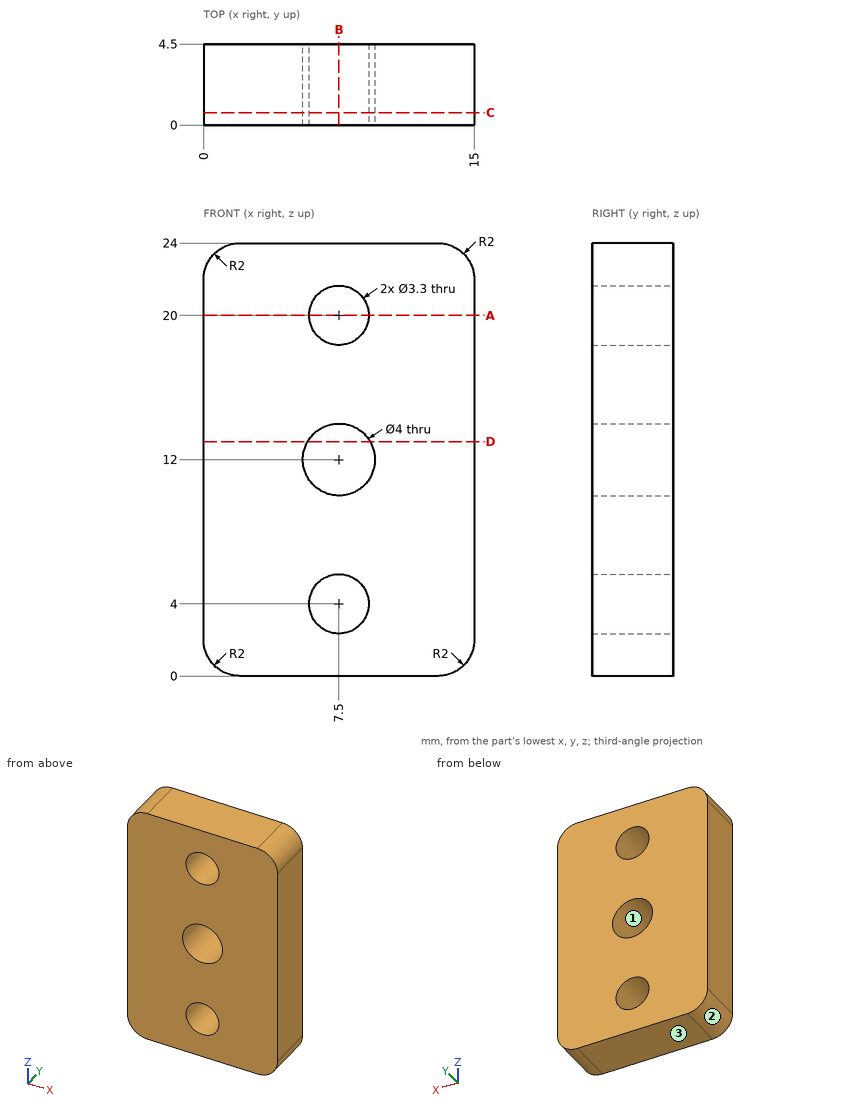
The drawing under review shows one solid part. Ordinate dimensions are in mm from its lowest x, y, z. Coordinates: 2 decimals unless noted, no trailing zeros. Write each loop counter-clockwise with the first axis right and the second up, starting at its lowest first coordinate (ties: lowest second). Pieces come first, ordered by that corner, then holes. Notation, with made-up numbers: (20.25, 71.5) - (50.25, 71.5) arc R17 cw to (50.25, 91.5) - close; hole circle Ø2 at (-11, 59). An arc over 180 degrees is marked (long way). Answer as CSV lines item,"result".
(1) We need section C-C (y = 0.7). Give the boundary of the cut face in (x, z), plus the area to 3 significant figures.
Data:
outline,"(0, 2) arc R2 ccw to (2, 0) - (13, 0) arc R2 ccw to (15, 2) - (15, 22) arc R2 ccw to (13, 24) - (2, 24) arc R2 ccw to (0, 22) - close; hole circle Ø4 at (7.5, 12); hole circle Ø3.3 at (7.5, 4); hole circle Ø3.3 at (7.5, 20)"
area,"327 mm2"
(2) We need section D-D (z = 13). Give the boundary of the cut face in (x, y).
Data:
outline,"(0, 0) - (5.77, 0) - (5.77, 4.5) - (0, 4.5) - close; (9.23, 0) - (15, 0) - (15, 4.5) - (9.23, 4.5) - close"
(3) We need section B-B (x = 7.5). Give the boundary of the cut face in (y, z).
Data:
outline,"(0, 0) - (4.5, 0) - (4.5, 2.35) - (0, 2.35) - close; (0, 5.65) - (4.5, 5.65) - (4.5, 10) - (0, 10) - close; (0, 14) - (4.5, 14) - (4.5, 18.35) - (0, 18.35) - close; (0, 21.65) - (4.5, 21.65) - (4.5, 24) - (0, 24) - close"
(4) Clearance check with flat-ended pins moving along their axes: pin 1 Ø1.5 at (x, y) = (12, 0.5) entering from -Z; pin 2 Ø2.5 at (x, z) = (7.5, 12) entering from +Y. State where each tip first meets the part, or that it passes through.
Data:
pin 1,"stops at z = 0"
pin 2,"passes through"
(5) Mouldability with a two-part tool opening along X and no side actions: class the marked faces 1, 2 and 3 as pulls with the +X half, pulls with the -X half, needs draft (parallel to the pull), parting line crosses it, or undercut.
Data:
face 1,"undercut"
face 2,"pulls with the -X half"
face 3,"needs draft"
(6) We need section A-A (z = 20). Give the boundary of the cut face in (x, y), plus the area to 4 significant figures.
Data:
outline,"(0, 0) - (5.85, 0) - (5.85, 4.5) - (0, 4.5) - close; (9.15, 0) - (15, 0) - (15, 4.5) - (9.15, 4.5) - close"
area,"52.65 mm2"
(7) For line 1 along Z through (x, y) = (7.5, 1.2); line 2 along Z through (x, y) = (8.75, 1.6); line 3 along X through (y, z) = (1.05, 12), list the stretches that pass through material, from the lowest coordinate up. Write a range as [from, to].
Data:
line 1,"z = [0, 2.35], [5.65, 10], [14, 18.35], [21.65, 24]"
line 2,"z = [0, 2.92], [5.08, 10.44], [13.56, 18.92], [21.08, 24]"
line 3,"x = [0, 5.5], [9.5, 15]"
